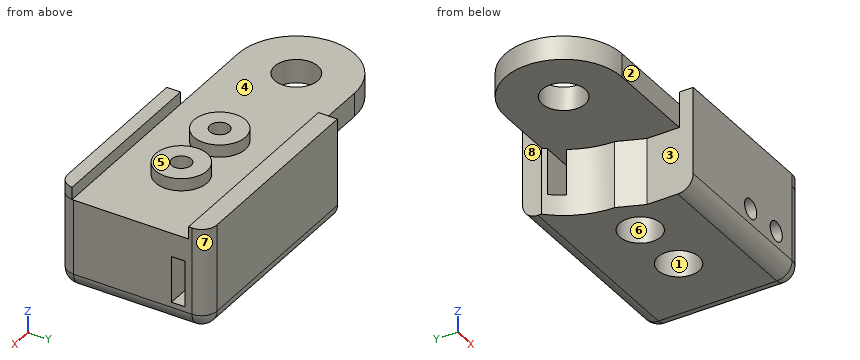
from build123d import *

# Parameters (mm, degrees)
BOSS_EXTRUDE1_DEPTH = 2
BOSS_EXTRUDE2_START = 4.5
BOSS_EXTRUDE2_DEPTH = 4.5
CUT_EXTRUDE1_DEPTH  = 4.5
BOSS_EXTRUDE3_DEPTH = 2.3
SKETCH9_R           = 2.1
CUT_EXTRUDE2_DEPTH  = 2.5
SKETCH10_R          = 2.5
BOSS_EXTRUDE4_DEPTH = 1.2
SKETCH11_R          = 0.95
CUT_EXTRUDE3_DEPTH  = 9.2
SKETCH12_R          = 2
CUT_EXTRUDE4_DEPTH  = 4.5
SKETCH14_W          = 20.343145751
SKETCH14_H          = 1.841510486
SKETCH14_W_2        = 17
SKETCH14_H_2        = 1.341637015
BOSS_EXTRUDE5_DEPTH = 1.2
FILLET1_R           = 1.5
SKETCH17_R          = 0.95
CUT_EXTRUDE5_DEPTH  = 3


# Read off the part's stored shape, not the designer's step: Boss-Extrude3
with BuildPart() as part:
    # Sketch5 → Boss-Extrude1 (new body)
    with BuildSketch(Plane.XY):
        with BuildLine():
            Line((8, 0), (9, -2.501635265))
            Line((9, -2.501635265), (9, -7.001635265))
            Line((9, -7.001635265), (26, -7.001635265))
            Line((26, -7.001635265), (26, 7.498364735))
            Line((26, 7.498364735), (5.656854249, 7.498364735))
            Line((5.656854249, 7.498364735), (5.656854249, 5.656854249))
            ThreePointArc((5.656854249, 5.656854249), (7.39103626, 3.061467459), (8, 0))
        make_face()
    extrude(amount=BOSS_EXTRUDE1_DEPTH)

    # Sketch6 → Boss-Extrude2 (add)
    with BuildSketch(Plane(origin=(0, 0, 0), x_dir=(-1, 0, 0), z_dir=(0, 0, -1)).offset(BOSS_EXTRUDE2_START)):
        with BuildLine():
            Line((-5.656854249, 7.498364735), (-5.656854249, 5.656854249))
            ThreePointArc((-5.656854249, 5.656854249), (-7.39103626, 3.061467459), (-8, 0))
            Line((-8, 0), (-9, -2.501635265))
            Line((-9, -2.501635265), (-9, -7.001635265))
            Line((-9, -7.001635265), (-26, -7.001635265))
            Line((-26, -7.001635265), (-26, 7.498364735))
            Line((-26, 7.498364735), (-5.656854249, 7.498364735))
        make_face()
    extrude(amount=-BOSS_EXTRUDE2_DEPTH)

    # Sketch7 → Cut-Extrude1 (cut)
    with BuildSketch(Plane(origin=(0, 0, -4.5), x_dir=(-1, 0, 0), z_dir=(0, 0, -1))):
        Polygon((-26, 5.298364735), (-2.738141148, 5.298364735), (-2.738141148, 3.998364735), (-29.849535112, 3.998364735), (-29.849535112, 5.298364735), align=None)
    extrude(amount=-CUT_EXTRUDE1_DEPTH, mode=Mode.SUBTRACT)

    # Boss-Extrude3 outline → Boss-Extrude3 (add)
    with BuildSketch(Plane(origin=(0, 0, -4.5), x_dir=(-1, 0, 0), z_dir=(0, 0, -1))):
        with BuildLine():
            Line((-9, -7.001635265), (-9, -5.65999825))
            Line((-9, -5.65999825), (0, -5.659997813))
            ThreePointArc((0, -5.659997813), (5.659997813, 0), (0, 5.659997813))
            Line((0, 5.659997813), (-5.656854249, 5.656854249))
            Line((-5.656854249, 5.656854249), (-5.656854249, 7.498364735))
            Line((-5.656854249, 7.498364735), (-26, 7.498364735))
            Line((-26, 7.498364735), (-26, -7.001635265))
            Line((-26, -7.001635265), (-9, -7.001635265))
        make_face()
    extrude(amount=BOSS_EXTRUDE3_DEPTH)

    # Sketch9 → Cut-Extrude2 (cut)
    with BuildSketch(Plane(origin=(0, 0, -6.8), x_dir=(-1, 0, 0), z_dir=(0, 0, -1))):
        Circle(SKETCH9_R)
    extrude(amount=-CUT_EXTRUDE2_DEPTH, mode=Mode.SUBTRACT)

    # Sketch10 → Boss-Extrude4 (add)
    with BuildSketch(Plane(origin=(0, 0, -6.8), x_dir=(-1, 0, 0), z_dir=(0, 0, -1))):
        with Locations((-12, 0)):
            Circle(SKETCH10_R)
        with Locations((-18, 0)):
            Circle(SKETCH10_R)
    extrude(amount=BOSS_EXTRUDE4_DEPTH)

    # Sketch11 → Cut-Extrude3 (cut)
    with BuildSketch(Plane(origin=(0, 0, -8), x_dir=(-1, 0, 0), z_dir=(0, 0, -1))):
        with Locations((-18, 0)):
            Circle(SKETCH11_R)
        with Locations((-12, 0)):
            Circle(SKETCH11_R)
    extrude(amount=-CUT_EXTRUDE3_DEPTH, mode=Mode.SUBTRACT)

    # Sketch12 → Cut-Extrude4 (cut)
    with BuildSketch(Plane.XY.offset(2)):
        with Locations((12, 0)):
            Circle(SKETCH12_R)
        with Locations((18, 0)):
            Circle(SKETCH12_R)
    extrude(amount=-CUT_EXTRUDE4_DEPTH, mode=Mode.SUBTRACT)

    # Sketch14 → Boss-Extrude5 (add)
    with BuildSketch(Plane(origin=(0, 0, -6.8), x_dir=(-1, 0, 0), z_dir=(0, 0, -1))):
        with Locations((-15.828427124, 6.577609492)):
            Rectangle(SKETCH14_W, SKETCH14_H)
        with Locations((-17.5, -6.330816758)):
            Rectangle(SKETCH14_W_2, SKETCH14_H_2)
    extrude(amount=BOSS_EXTRUDE5_DEPTH)

    # Fillet1
    # the kernel refuses this fillet: 1.5 mm, written as the material it takes off along each edge
    with BuildSketch(Plane(origin=(24.5, -5.501635265, 0.5), x_dir=(0, 0, 1), z_dir=(0, -1, 0))) as fillet1_piece_1_section:
        Polygon((0, 0), (FILLET1_R, 0), (FILLET1_R, -FILLET1_R), (0, -FILLET1_R), align=None)
    fillet1_piece_1 = extrude(amount=FILLET1_R, mode=Mode.PRIVATE)
    fillet1_piece_1 = fillet1_piece_1 - Plane(origin=(24.5, -5.501635265, 0.5), x_dir=(-0.7071067811865475, 0, -0.7071067811865475), z_dir=(0, -1, 0)) * Sphere(FILLET1_R, mode=Mode.PRIVATE)
    add(fillet1_piece_1, mode=Mode.SUBTRACT)
    with BuildSketch(Plane(origin=(24.5, 5.998364735, 0.5), x_dir=(0, 0, 1), z_dir=(0, 1, 0))) as fillet1_piece_2_section:
        Polygon((0, 0), (FILLET1_R, 0), (FILLET1_R, FILLET1_R), (0, FILLET1_R), align=None)
    fillet1_piece_2 = extrude(amount=FILLET1_R, mode=Mode.PRIVATE)
    fillet1_piece_2 = fillet1_piece_2 - Plane(origin=(24.5, 5.998364735, 0.5), x_dir=(-0.7071067811865475, 0, -0.7071067811865475), z_dir=(0, 1, 0)) * Sphere(FILLET1_R, mode=Mode.PRIVATE)
    add(fillet1_piece_2, mode=Mode.SUBTRACT)
    with BuildSketch(Plane(origin=(26, -5.501635265, 2), x_dir=(-1, 0, 0), z_dir=(0, 1, 0))) as fillet1_piece_3:
        with BuildLine():
            CenterArc((FILLET1_R, -FILLET1_R), FILLET1_R, 90, 90)
            Line((0, -FILLET1_R), (0, 0))
            Line((0, 0), (FILLET1_R, 0))
        make_face()
    extrude(amount=11.5, mode=Mode.SUBTRACT)
    with BuildSketch(Plane(origin=(26, -7.001635265, -4.5), x_dir=(-1, 0, 0), z_dir=(0, 0, 1))) as fillet1_piece_4:
        with BuildLine():
            CenterArc((FILLET1_R, -FILLET1_R), FILLET1_R, 90, 90)
            Line((0, -FILLET1_R), (0, 0))
            Line((0, 0), (FILLET1_R, 0))
        make_face()
    extrude(amount=5, mode=Mode.SUBTRACT)
    with BuildSketch(Plane(origin=(5.25, -7.001635265, 2), x_dir=(0, 1, 0), z_dir=(1, 0, 0))) as fillet1_piece_5:
        with BuildLine():
            CenterArc((FILLET1_R, -FILLET1_R), FILLET1_R, 90, 90)
            Line((0, -FILLET1_R), (0, 0))
            Line((0, 0), (FILLET1_R, 0))
        make_face()
    extrude(amount=19.25, mode=Mode.SUBTRACT)
    with BuildSketch(Plane(origin=(24.5, 7.498364735, 2), x_dir=(0, -1, 0), z_dir=(-1, 0, 0))) as fillet1_piece_6:
        with BuildLine():
            CenterArc((FILLET1_R, -FILLET1_R), FILLET1_R, 90, 90)
            Line((0, -FILLET1_R), (0, 0))
            Line((0, 0), (FILLET1_R, 0))
        make_face()
    extrude(amount=22.593145751, mode=Mode.SUBTRACT)
    with BuildSketch(Plane(origin=(26, 7.498364735, -4.5), x_dir=(-1, 0, 0), z_dir=(0, 0, 1))) as fillet1_piece_7:
        with BuildLine():
            CenterArc((FILLET1_R, FILLET1_R), FILLET1_R, 180, 90)
            Line((0, FILLET1_R), (0, 0))
            Line((0, 0), (FILLET1_R, 0))
        make_face()
    extrude(amount=5, mode=Mode.SUBTRACT)
    with BuildSketch(Plane(origin=(26, 7.498364735, -4.5), x_dir=(-1.0, -1.9174232572065026e-10, 0), z_dir=(0, 0, -1))) as fillet1_piece_8:
        with BuildLine():
            CenterArc((FILLET1_R, -FILLET1_R), FILLET1_R, 90.000000011, 90)
            Line((FILLET1_R * 1.9173522033e-10, -FILLET1_R), (0, 0))
            Line((0, 0), (FILLET1_R, 0))
        make_face()
    extrude(amount=2.3, mode=Mode.SUBTRACT)
    with BuildSketch(Plane(origin=(26, 7.498364735, -6.8), x_dir=(-1, 0, 0), z_dir=(0, 0, -1))) as fillet1_piece_9:
        with BuildLine():
            CenterArc((FILLET1_R, -FILLET1_R), FILLET1_R, 90, 90)
            Line((0, -FILLET1_R), (0, 0))
            Line((0, 0), (FILLET1_R, 0))
        make_face()
    extrude(amount=4.95, mode=Mode.SUBTRACT)
    with BuildSketch(Plane(origin=(26, -7.001635265, -4.5), x_dir=(-1.0, -1.9169850891861218e-10, 0), z_dir=(0, 0, -1))) as fillet1_piece_10:
        with BuildLine():
            CenterArc((FILLET1_R, FILLET1_R), FILLET1_R, 180.000000011, 90)
            Line((-FILLET1_R * 1.91707982785e-10, FILLET1_R), (0, 0))
            Line((0, 0), (FILLET1_R, 0))
        make_face()
    extrude(amount=2.3, mode=Mode.SUBTRACT)
    with BuildSketch(Plane(origin=(26, -7.001635265, -6.8), x_dir=(-1, 0, 0), z_dir=(0, 0, -1))) as fillet1_piece_11:
        with BuildLine():
            CenterArc((FILLET1_R, FILLET1_R), FILLET1_R, 180, 90)
            Line((0, FILLET1_R), (0, 0))
            Line((0, 0), (FILLET1_R, 0))
        make_face()
    extrude(amount=4.95, mode=Mode.SUBTRACT)

    # Sketch17 → Cut-Extrude5 (cut)
    with BuildSketch(Plane.XZ.offset(7.001635265)):
        with Locations((22, -1)):
            Circle(SKETCH17_R)
        with Locations((18, -1)):
            Circle(SKETCH17_R)
    extrude(amount=-CUT_EXTRUDE5_DEPTH, mode=Mode.SUBTRACT)

    # Mirror1: part across plane


with BuildPart() as part_1:
    add(part.part)
    add(part.part.mirror(Plane(origin=(0, 0, -8), x_dir=(1, 0, 0), z_dir=(0, 0, -1))))


with BuildPart() as body_2:
    # Split1: the piece on the far side of the plane
    add(part_1.part)
    split(bisect_by=Plane(origin=(0, 0, -8), x_dir=(-1, 0, 0), z_dir=(0, 0, -1)), keep=Keep.BOTTOM)


with BuildPart() as part_2:
    add(part_1.part)

    # Split1
    split(bisect_by=Plane(origin=(0, 0, -8), x_dir=(-1, 0, 0), z_dir=(0, 0, -1)), keep=Keep.TOP)


solid = part_2.part
Can you work these out from the model? Positions are in its coordinate system, mm. Face numbers are marked on the shaded views. A direction names the side the tool comes from. Round coordinates to 2 decimals unless told otherwise and drop trailing zeros. Loops run counter-clockwise (first coordinate to the right, second up) from the corner with the lowest first, then second, coordinate; pieces in that order, holes last. Notation, with made-up numbers: (-40, 49) - (-27, 49) arc R21 ccw to (-27, 88) - close; hole circle Ø6 at (87.5, 9.25). An arc over 180 degrees is marked (long way). Answer in a Markdown table with one row per item. Add a question column.
Q1. I want a section at D-D on x = 22. List the corners of the cut face in (y, z) for me.
Q2. I want a section at A-A on z = -15. List the corners of the cut face in (x, y) for me, and give its area (3 significant figures).
Q3. I want a section at B-B on x = 12. List the corners of the cut face in (y, z) for me.
Q4. I need wall thicknesses on L1, parallel to Y at x = 12, z = -8.25; L2, parallel to Y at x = 14, z = -12.25; L3, parallel to X at y = -5.1, z = -15. Which ranges of each line are inside material? Lowest first, please.
Q5. I want a section at C-C on z = -11. List the corners of the cut face in (x, y) for me.
Q6. Which directions (+Z, -Z, +X, -X, +Y, -Y) give clear straight access to the entire face, cutting with the end or side of a thin tool? Please do the marked faces 1, 2, 3 and 4.
Q7. For pin 1 Ø0.9 at (y, z) = (6.5, -11.5) entering from -X; pin 2 Ø5 at (x, y) = (-0.5, 3) entering from +Z; pin 3 Ø1.2 at (x, y) = (11.5, 0.5) entering from -Z, each with a flat end and sliding along its axis, tell me the tip position at first contact or that it passes through.
Q8. We'd pull the mould along X, two halves only. Please class the marked faces 5, 6, 7 and 8: pulls with the +X half, pulls with the -X half, needs draft (parallel to the pull), parting line crosses it, or undercut.
A:
| question | item | result |
|---|---|---|
| 1 | outline | (-7, -16.5) arc R1.5 ccw to (-5.5, -18) - (6, -18) arc R1.5 ccw to (7.5, -16.5) - (7.5, -8) - (5.66, -8) - (5.66, -9.2) - (-5.66, -9.2) - (-5.66, -8) - (-7, -8) - (-7, -14.05) - (-4, -14.05) - (-4, -15.95) - (-7, -15.95) - close; hole (4, -16) - (5.3, -16) - (5.3, -11.5) - (4, -11.5) - close |
| 2 | outline | (5.66, 5.66) arc R8 cw to (5.99, 5.3) - (26, 5.3) - (26, 6) arc R1.5 ccw to (24.5, 7.5) - (5.66, 7.5) - close; (6.93, 4) arc R8 cw to (8, 0) - (9, -2.5) - (9, -7) - (17.05, -7) - (17.05, -4) - (18.95, -4) - (18.95, -7) - (21.05, -7) - (21.05, -4) - (22.95, -4) - (22.95, -7) - (24.5, -7) arc R1.5 ccw to (26, -5.5) - (26, 4) - close; hole circle Ø4 at (12, 0); hole circle Ø4 at (18, 0) |
| 2 | area | 201 mm^2 |
| 3 | outline | (-7, -16.5) arc R1.5 ccw to (-5.5, -18) - (-2, -18) - (-2, -13.5) - (-0.95, -13.5) - (-0.95, -8) - (-2.5, -8) - (-2.5, -9.2) - (-5.66, -9.2) - (-5.66, -8) - (-7, -8) - close; (0.95, -13.5) - (2, -13.5) - (2, -18) - (6, -18) arc R1.5 ccw to (7.5, -16.5) - (7.5, -8) - (5.66, -8) - (5.66, -9.2) - (2.5, -9.2) - (2.5, -8) - (0.95, -8) - close; hole (4, -16) - (5.3, -16) - (5.3, -11.5) - (4, -11.5) - close |
| 4 | L1 | -7 to -5.66, -2.5 to -0.95, 0.95 to 2.5, 5.66 to 7.5 |
| 4 | L2 | -7 to 4, 5.3 to 7.5 |
| 4 | L3 | 9 to 17.05, 18.95 to 21.05, 22.95 to 26 |
| 5 | outline | (0, -5.66) - (9, -5.66) - (9, -7) - (24.5, -7) arc R1.5 ccw to (26, -5.5) - (26, 6) arc R1.5 ccw to (24.5, 7.5) - (5.66, 7.5) - (5.66, 5.66) - (0, 5.66) arc R5.66 ccw to start; hole circle Ø4.2 at (0, 0); hole circle Ø1.9 at (12, 0); hole circle Ø1.9 at (18, 0) |
| 6 | face 1 | -Z |
| 6 | face 2 | +Z, -Z, -X, -Y |
| 6 | face 3 | -Z, -X, -Y |
| 6 | face 4 | +Z |
| 7 | pin 1 | x = 5.66 |
| 7 | pin 2 | z = -9.2 |
| 7 | pin 3 | z = -13.5 |
| 8 | face 5 | needs draft |
| 8 | face 6 | undercut |
| 8 | face 7 | pulls with the +X half |
| 8 | face 8 | pulls with the -X half |
